Could you check a few things on this model? Use its own coordinates, in mm. Coordinates: 2 decimals unless noted, no trailing zeros. Write each loop counter-clockwise with the first axis right and the second up, starting at its lowest first coordinate (ties: lowest second). Pieces come first, ordered by that corner, then holes.
Autodesk Inventor part; units mm, degrees
ref_plane "YZ Plane" through (0, 0, 0) normal (1, 0, 0) x (0, 1, 0)
ref_plane "XZ Plane" through (0, 0, 0) normal (0, 1, 0) x (-1, 0, 0)
ref_plane "XY Plane" through (0, 0, 0) normal (0, 0, 1) x (1, 0, 0)
sketch "Sketch1" plane through (0, 0, 0) normal (0, 0, 1) x (1, 0, 0)
  line L0 (-44, -28) -> (44, -28)
  line L1 (44, -28) -> (44, 28)
  line L2 (44, 28) -> (-44, 28)
  line L3 (-44, 28) -> (-44, -28)
  line L4 (-44, -28) -> (44, 28) construction
  line L5 (44, -28) -> (-44, 28) construction
  point P0 (0, 0)
  dimension "d0" = 88
  dimension "d1" = 56
extrude "Extrusion1" add sketch "Sketch1" along normal blind 3
fillet "Fillet1" radius 2 4 edges at (44, 28, 1.5) (44, -28, 1.5) (-44, 28, 1.5) (-44, -28, 1.5)
sketch "Sketch2" plane through (0, 0, 3) normal (0, 0, 1) x (1, 0, 0)
  line L0 (-40.5, -24.5) -> (40.5, -24.5)
  line L1 (40.5, -24.5) -> (40.5, 24.5)
  line L2 (40.5, 24.5) -> (-40.5, 24.5)
  line L3 (-40.5, 24.5) -> (-40.5, -24.5)
  line L4 (-40.5, -24.5) -> (40.5, 24.5) construction
  line L5 (40.5, -24.5) -> (-40.5, 24.5) construction
  point P0 (0, 0)
  point P1 (-40.5, 24.5)
  dimension "d12" = 81
  dimension "d13" = 49
hole "Hole1" at (-40.5, -24.5, 3) at (-40.5, 24.5, 3) at (40.5, -24.5, 3) at (40.5, 24.5, 3) direction (0, 0, -1) diameter 3 end through all
properties part number "Distance_plate"
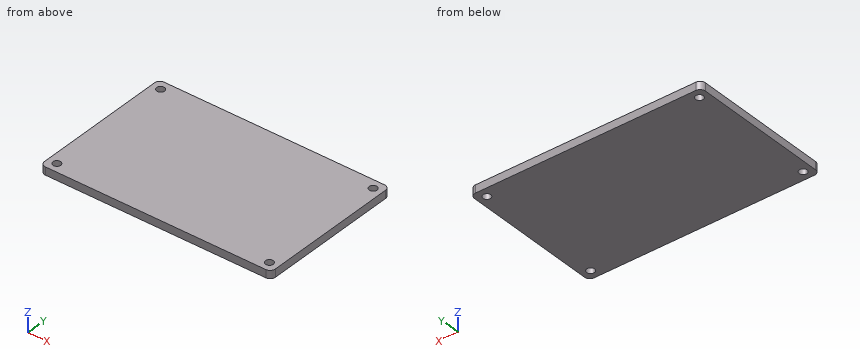
1. I want a section at A-A on x = 40.5. Please give me the cut outline in (y, z), plus the area to 3 significant figures.
Verdict:
outline: (-28, 0) - (-26, 0) - (-26, 3) - (-28, 3) - close; (-23, 0) - (23, 0) - (23, 3) - (-23, 3) - close; (26, 0) - (28, 0) - (28, 3) - (26, 3) - close
area: 150 mm2
2. Please list where these lines run through material, in increasing order: line 1 along Y through (x, z) = (-40.5, 0.85); line 2 along X through (y, z) = (24.5, 1.5); line 3 along X through (y, z) = (-25, 0.25).
Verdict:
line 1: y = -28 to -26, -23 to 23, 26 to 28
line 2: x = -44 to -42, -39 to 39, 42 to 44
line 3: x = -44 to -41.91, -39.09 to 39.09, 41.91 to 44
3. I want a section at B-B on y = 24.5. Please give me the cut outline in (x, z), plus the area to 3 significant figures.
Verdict:
outline: (-44, 0) - (-42, 0) - (-42, 3) - (-44, 3) - close; (-39, 0) - (39, 0) - (39, 3) - (-39, 3) - close; (42, 0) - (44, 0) - (44, 3) - (42, 3) - close
area: 246 mm2
